Source: CAD feature listing. Evaluate the final solid. Frame: model axes, mm. Face numbers are marked on the shaded views. A direction names the side the tool comes from. Coordinates: 2 decimals unless noted, no trailing zeros. Order: outer loops, then holes, each group sorted by start corner. A loop starts at its lowest first (then second) coordinate and runs counter-clockwise, first axis right, second up. Notation, with made-up numbers: (13, -39) - (50, -39) arc R12 cw to (50, -16) - close; hole circle Ø2 at (69.25, 73.25). An arc over 180 degrees is marked (long way). One line per question, with ' | ' between items.
from build123d import *

# Parameters (mm, degrees)
F2_R = 1.9622727835


with BuildPart() as f1:
    # F0 (on Top) → F1 (revolve)
    with BuildSketch(Plane.XY):
        Polygon((-21.0659306824, -27.7770664543), (-21.0659306824, 15.4031372249), (-21.0659306824, 28.1031372249), (-24.4244831643, 28.1031372249), (-27.0358305424, 20.7487531006), (-27.0358305424, -27.7770664543), align=None)
        Polygon((-24.4244831643, 28.1031372249), (-21.0659306824, 28.1031372249), (-21.0659306824, 43.5661226511), (-24.4244831643, 43.5661226511), (-24.4244831643, 41.9496893883), align=None)
        with BuildLine():
            ThreePointArc((-24.4244831643, 43.5661226511), (-24.9002133782, 42.7579060197), (-24.4244831643, 41.9496893883))
            Line((-24.4244831643, 41.9496893883), (-24.4244831643, 43.5661226511))
        make_face()
    revolve(axis=Axis((-21.0659306824, -6.1869646147, 0), (0, -1, 0)))

    # F2
    f2_edges = [f1.edges().sort_by_distance(p)[0] for p in [
        (-15.096031, -27.777066, 0),
    ]]
    fillet(f2_edges, radius=F2_R)


solid = f1.part
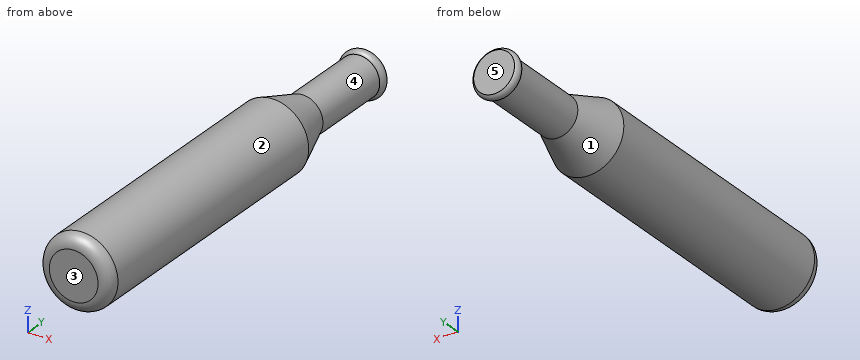
(1) Cut plane A-A (z = 0). Return the cut outline in (x, y), and give its area (3 significant figures).
Taken from the geometry:
outline: (-27.04, -25.81) arc R1.96 ccw to (-25.07, -27.78) - (-17.06, -27.78) arc R1.96 ccw to (-15.1, -25.81) - (-15.1, 20.75) - (-17.71, 28.1) - (-17.71, 41.95) arc R0.92 ccw to (-17.71, 43.57) - (-24.42, 43.57) arc R0.92 ccw to (-24.42, 41.95) - (-24.42, 28.1) - (-27.04, 20.75) - close | area: 751 mm²
(2) Pull-direction query (Y, two-part tool) for the marked faces 3, 4 and 5; classes: pulls with the +Y half, pulls with the -Y half, needs draft (parallel to the pull), parting line crosses it, or undercut.
Taken from the geometry:
face 3: pulls with the -Y half | face 4: undercut | face 5: pulls with the +Y half
(3) Cut plane B-B (y = 31). Return the cut outline in (x, z).
Taken from the geometry:
outline: circle Ø6.72 at (-21.07, 0)
(4) Material intervals for L1, parallel to Z at x = -25.5, y = 10.5; L2, parallel to Z at x = -21.25, y = 16; L3, parallel to X at y = 4.5, z = 3.75, sorted ascending. Write a range as from..to.
Taken from the geometry:
L1: z = -4..4 | L2: z = -5.97..5.97 | L3: x = -25.71..-16.42
(5) Pin query (flat end, axial travel): P1, Ø1, axis at x = -24, y = 19, coming from the -Z side; P2, Ø5, axis at y = 6.5, z = -3, coming from the -X side. Return the tip coordinate at first contact, or that it passes through.
Taken from the geometry:
P1: stops at z = -5.45 | P2: stops at x = -27.01
(6) Cut plane C-C (y = 1). Return the cut outline in (x, z).
Taken from the geometry:
outline: circle Ø11.94 at (-21.07, 0)
(7) Set-up query: the marked faces 1 and 2. Return all of +Z, -Z, +X, -X, +Y, -Y with unobstructed straight access to the full face (end or side cutting, diameter ignored); none if empty.
Taken from the geometry:
face 1: none | face 2: +Y, -Y
